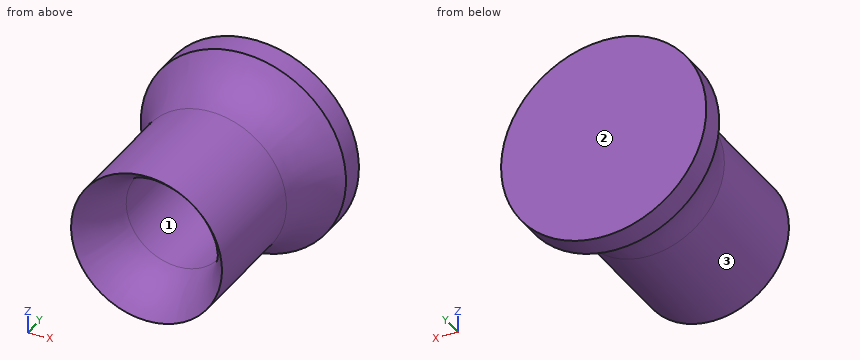
from build123d import *

# Parameters (mm, degrees)
SKETCH1_R           = 12.699999999999998
BOSS_EXTRUDE1_DEPTH = 25.4
SKETCH2_R           = 6.34
CUT_EXTRUDE1_DEPTH  = 22.4
SKETCH3_R           = 12.7
SKETCH3_R_2         = 9.340000000000002
CUT_EXTRUDE4_DEPTH  = 22.4
FILLET1_R           = 10


with BuildPart() as part:
    # Sketch1 → Boss-Extrude1 (new body)
    with BuildSketch(Plane(origin=(0, 0, 0), x_dir=(1, 0, 0), z_dir=(0, 1, 0))):
        with Locations(Location((0, 0, 0), (0, 0, 270))):
            Circle(SKETCH1_R)
    extrude(amount=BOSS_EXTRUDE1_DEPTH)

    # Sketch2 → Cut-Extrude1 (cut)
    with BuildSketch(Plane.XZ):
        with Locations(Location((0, 0, 0), (0, 0, 270))):
            Circle(SKETCH2_R)
    extrude(amount=-CUT_EXTRUDE1_DEPTH, mode=Mode.SUBTRACT)

    # Sketch3 → Cut-Extrude4 (cut)
    with BuildSketch(Plane.XZ):
        with Locations(Location((0, 0, 0), (0, 0, 90))):
            Circle(SKETCH3_R)
        with Locations(Location((0, 0, 0), (0, 0, 270))):
            Circle(SKETCH3_R_2, mode=Mode.SUBTRACT)
    extrude(amount=-CUT_EXTRUDE4_DEPTH, mode=Mode.SUBTRACT)

    # Fillet1
    # the kernel refuses this fillet: 10 mm, written as the material it adds along each edge
    with BuildSketch(Plane(origin=(0, 22.4, 0), x_dir=(-1.8e-16, 0, -1), z_dir=(-1, 0, 1.8e-16))) as fillet1_piece_1:
        with BuildLine():
            CenterArc((19.340000000000003, 7.477325725150667), FILLET1_R, 180, 48.39434621608348)
            Line((9.340000000000003, 7.477325725150667), (9.140000000000004, 7.477325725150667))
            Line((9.140000000000004, 7.477325725150667), (9.140000000000002, 0))
            Line((9.140000000000002, 0), (9.340000000000002, -0.1999999999999993))
            ThreePointArc((9.340000000000002, -0.1999999999999993), (11.02, -0.1999999999999993), (12.5672, -0.1495465145030117))
            Line((12.5672, -0.1495465145030117), (12.7, 0))
        make_face()
    revolve(axis=Axis((0, 22.4, 0), (0, -1, 0)))
    # the kernel refuses this fillet: 10 mm, written as the material it takes off along each edge
    with BuildSketch(Plane(origin=(0, 0, 0), x_dir=(-1.8e-16, 0, -1), z_dir=(-1, 0, 1.8e-16))) as fillet1_2_piece_1:
        with BuildLine():
            CenterArc((16.339999999999996, -7.141428428542857), FILLET1_R, 134.42700400080568, 45.57299599919432)
            Line((6.339999999999996, -7.141428428542857), (6.139999999999996, -7.141428428542857))
            Line((6.139999999999996, -7.141428428542857), (6.14, 0))
            Line((6.14, 0), (6.34, 0.2))
            ThreePointArc((6.34, 0.2), (7.840000000000001, 0.2), (9.200000000000001, 0.14282856857085713))
            Line((9.200000000000001, 0.14282856857085713), (9.340000000000002, 0))
        make_face()
    revolve(axis=Axis((0, 0, 0), (0, -1, 0)), mode=Mode.SUBTRACT)


solid = part.part
Part model, mm, in its own coordinate system. Face numbers are marked on the shaded views. Coordinates: 2 decimals unless noted, no trailing zeros. Write each loop counter-clockwise with the first axis right and the second up, starting at its lowest first coordinate (ties: lowest second). Pieces come first, ordered by that corner, then holes. Notation, with made-up numbers: M 70,70.5 L 99,70.5 A10 cw 99,80.5 Z; hole C 45,50 d5. An arc over 180 degrees is marked long. Return JSON: item names as keys, results as strings.
1. Saw through at A-A, the plane z = 0. Write the cut outline in (x, y), then the cut area to 3 significant figures.
Determined:
{"outline": "M -12.7,22.4 A10 cw -9.34,14.92 L -9.34,0 A10 ccw -6.34,7.14 L -6.34,22.4 L 6.34,22.4 L 6.34,7.14 A10 ccw 9.34,0 L 9.34,14.92 A10 cw 12.7,22.4 L 12.7,25.4 L -12.7,25.4 Z", "area": "213 mm²"}
2. Saw through at B-B, the plane x = 0. Write the cut outline in (y, z), then the cut area to 3 significant figures.
Determined:
{"outline": "M 0,-9.34 L 14.92,-9.34 A10 cw 22.4,-12.7 L 25.4,-12.7 L 25.4,12.7 L 22.4,12.7 A10 cw 14.92,9.34 L 0,9.34 A10 ccw 7.14,6.34 L 22.4,6.34 L 22.4,-6.34 L 7.14,-6.34 A10 ccw Z", "area": "213 mm²"}
3. Saw through at C-C, the plane y = 10.75. Write the cut outline in (x, z).
Determined:
{"outline": "C 0,0 d18.68; hole C 0,0 d12.68"}
4. Saw through at D-D, the plane y = 20. Write the cut outline in (x, z).
Determined:
{"outline": "C 0,0 d21.45; hole C 0,0 d12.68"}
5. Probe L1, parallel to X at y = 14.5, z = 0; L2, parallel to X at y = 6, z = 1.75; L3, parallel to Z at x = -4, y = 10.25. List the from-to ranges inside material, lowest first.
Determined:
{"L1": "-9.34 to -6.34, 6.34 to 9.34", "L2": "-9.17 to -6.16, 6.16 to 9.17", "L3": "-8.44 to -4.92, 4.92 to 8.44"}
6. Flat gauge pins, fed straight in: pin 1 Ø1.5 at (x, y) = (-1, 5.5) entering from -Z; pin 2 Ø2 at (y, z) = (10, -8) entering from -X; pin 3 Ø1.5 at (y, z) = (14, -2.5) entering from -X. Where does each tip first touch, or does it go through?
Determined:
{"pin 1": "z = -9.34", "pin 2": "x = -6.18", "pin 3": "x = -9.17"}
7. Pull direction Z, two halves, no side cores. Call the marked faces 1, 2 and 3: pulls with the +Z half, pulls with the -Z half, needs draft (parallel to the pull), parting line crosses it, or undercut.
Determined:
{"face 1": "undercut", "face 2": "needs draft", "face 3": "parting line crosses it"}
